Verification items for this drawing (mm, ordinates from the low corner). Give positions to 0.01 mm unless a question says otherwise; leave off trailing zeros. Loops run counter-clockwise (first coordinate to the right, second up) from the corner with the lowest first, then second, coordinate; pieces in that order, holes last. Notation, with made-up numbers: (2.25, 24.25) -> (53.25, 24.25) arc R28 ccw to (53.25, 45.25) -> close; hole circle Ø11 at (-39.75, -25). An arc over 180 degrees is marked (long way). Write each question's results on one line, items separated by ' | '. Start each with the question number.
Item 1: Cross-section at A-A on y = 21.25. Enter the section's corners in (x, z) (3 decimals), then the cut area to 3 significant figures.
Item 2: Gauge pin test, flat ends, axial feed: pin 1 Ø12 at (x, z) = (23, 46.5) entering from -Y; pin 2 Ø1.5 at (y, z) = (29, 63) entering from +X; pin 3 Ø2 at (x, z) = (20.5, 64) entering from +Y; pin 4 Ø4 at (x, y) = (21.25, 21.25) entering from -Z. Record the tip position at first contact, or that the pin passes through.
Item 3: Cross-section at B-B on z = 59. Enter the section's corners in (x, y) (3 decimals).
Item 4: Mould release check, pull along X, two halves, no side actions. Record for the marked faces 1, 2, 3 and 4: pulls with the +X half, pulls with the -X half, needs draft (parallel to the pull), parting line crosses it, or undercut.
Item 5: Scan lines: line 1 along Y through (x, z) = (21.25, 47.5) (3 decimals); line 2 along X through (y, z) = (21, 28); line 3 along Y through (x, z) = (24, 11). Record each from-to range of solid material in increasing order.
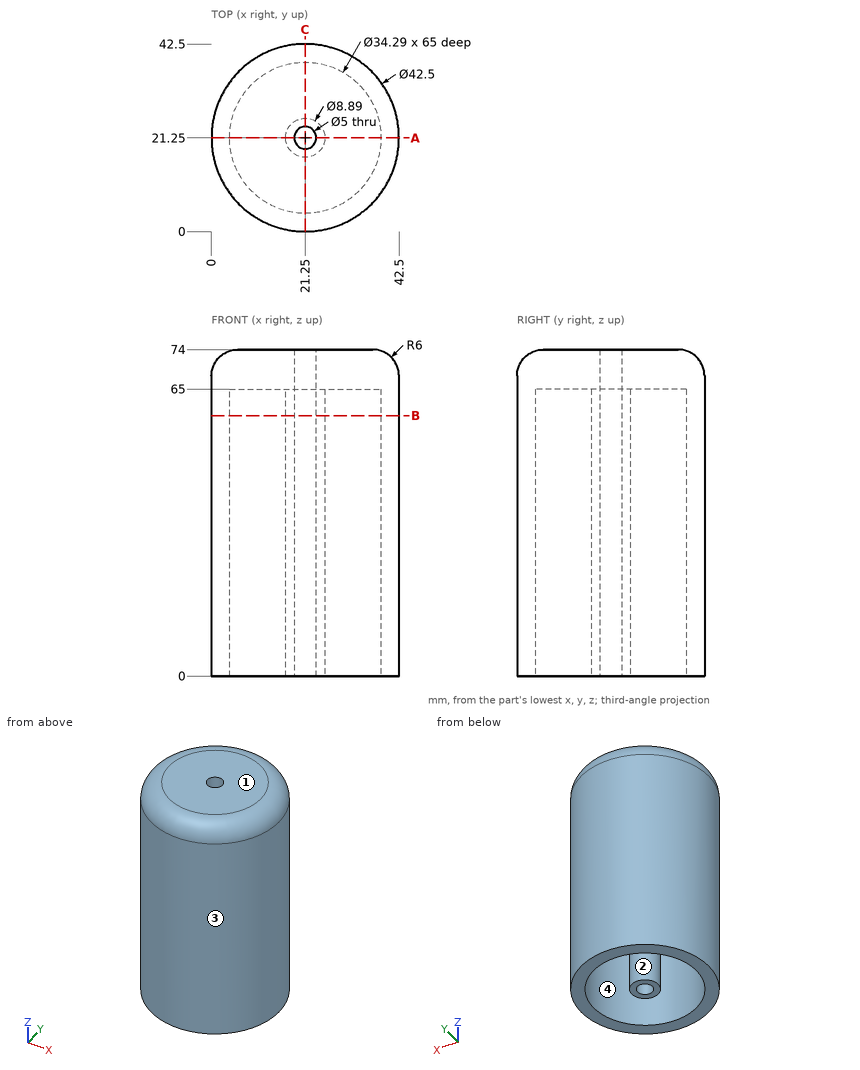
Answer sheet:
1) outline: (0, 0) -> (4.105, 0) -> (4.105, 65) -> (16.805, 65) -> (16.805, 0) -> (18.75, 0) -> (18.75, 74) -> (6, 74) arc R6 ccw to (0, 68) -> close; (23.75, 0) -> (25.695, 0) -> (25.695, 65) -> (38.395, 65) -> (38.395, 0) -> (42.5, 0) -> (42.5, 68) arc R6 ccw to (36.5, 74) -> (23.75, 74) -> close | area: 1,110 mm²
2) pin 1: stops at y = 0 | pin 2: stops at x = 41.31 | pin 3: stops at y = 42.5 | pin 4: passes through
3) outline: circle Ø42.5 at (21.25, 21.25); circle Ø8.89 at (21.25, 21.25); hole circle Ø34.29 at (21.25, 21.25); hole circle Ø5 at (21.25, 21.25)
4) face 1: needs draft | face 2: undercut | face 3: parting line crosses it | face 4: undercut
5) line 1: y = 0 to 4.105, 16.805 to 18.75, 23.75 to 25.695, 38.395 to 42.5 | line 2: x = 0 to 4.11, 16.81 to 18.76, 23.74 to 25.69, 38.39 to 42.5 | line 3: y = 0.18 to 4.33, 17.76 to 24.74, 38.17 to 42.32
